from build123d import *

# Parameters (mm, degrees)
F0_R      = 2.25
F1_DEPTH  = 10
F3_DEPTH  = 20
F4_R      = 2.01
F5_DEPTH  = 5
F6_R      = 2.25
F7_DEPTH  = 5
F8_R      = 3.75
F9_DEPTH  = 2
F10_R     = 3.75
F11_DEPTH = 2


with BuildPart() as f1:
    # F0 (on Top) → F1 (new body)
    with BuildSketch(Plane.XY):
        Polygon((15.558824, 6.264706), (15.558824, -35.735294), (35.558824, -35.735294), (35.558824, -13.735294), (55.558824, 6.264706), (120.558824, 6.264706), (120.558824, 26.264706), (35.558824, 26.264706), (35.558824, 6.264706), align=None)
        with Locations((25.558824, -20.735294)):
            Circle(F0_R, mode=Mode.SUBTRACT)
        with Locations((25.558824, -5.735294)):
            Circle(F0_R, mode=Mode.SUBTRACT)
        with Locations((54.558824, 16.264706)):
            Circle(F0_R, mode=Mode.SUBTRACT)
        with Locations((109.558824, 16.264706)):
            Circle(F0_R, mode=Mode.SUBTRACT)
    extrude(amount=F1_DEPTH)

    # F2 (on face) → F3 (join)
    with BuildSketch(Plane.XY.offset(10)):
        Polygon((55.558824, 6.264706), (35.558824, 6.264706), (35.558824, -13.735294), (40.558824, -8.735294), (40.558824, 1.264706), (45.558824, 1.264706), (50.558824, 1.264706), align=None)
    extrude(amount=F3_DEPTH)

    # F4 (on face) → F5 (cut)
    with BuildSketch(Plane(origin=(35.558824, 0, 0), x_dir=(0, -1, 0), z_dir=(-1, 0, 0))):
        with Locations((6.735294, 20)):
            Circle(F4_R)
    extrude(amount=-F5_DEPTH, mode=Mode.SUBTRACT)

    # F6 (on face) → F7 (cut)
    with BuildSketch(Plane(origin=(0, 6.264706, 0), x_dir=(-1, 0, 0), z_dir=(0, 1, 0))):
        with Locations((-48.558824, 20)):
            Circle(F6_R)
    extrude(amount=-F7_DEPTH, mode=Mode.SUBTRACT)

    # F8 (on face) → F9 (cut)
    with BuildSketch(Plane.XZ.offset(-1.264706)):
        with Locations((48.558824, 20)):
            Circle(F8_R)
    extrude(amount=-F9_DEPTH, mode=Mode.SUBTRACT)

    # F10 (on face) → F11 (cut)
    with BuildSketch(Plane.YZ.offset(40.558824)):
        with Locations((-6.735294, 20)):
            Circle(F10_R)
    extrude(amount=-F11_DEPTH, mode=Mode.SUBTRACT)


solid = f1.part
Source: CAD feature listing. Evaluate the final solid. Frame: model axes, mm. A direction names the side the tool comes from. Round coordinates to 2 decimals unless told otherwise and drop trailing zeros. Loops run counter-clockwise (first coordinate to the right, second up) from the corner with the lowest first, then second, coordinate; pieces in that order, holes last.
Q1. Ray query, line 1 (X direction, y = 2.5, z = 20); line 2 (X direction, y = -2.5, z = 21.5); line 3 (Y direction, x = 42, z = 22). Return the intervals inside material, ascending.
Q2. Mould query, pull axis Y, two halves, no side actions, for faces 1 (the face through (50, 3.265, 18)), 2 (the face through (23.31, -5.64, 4.93)), 3 (the face through (37.038, -6.474, 21.993)), 4 (the face through (77, 16, 10)). Classes: pulls with the +Y half, pulls with the -Y half, needs draft (parallel to the pull), parting line crosses it, or undercut.
Q3. First-contact query: P1, Ø6, axis at y = -6.74, z = 20, coming from the -X side; P2, Ø10, axis at x = 42, y = 15.5, coming from the +Z side; P3, Ø11, axis at y = -5, z = 16, coming from the +X side. Flat tips, straight axial feed; report the tip coordinate or a pass-through.
Q4. Section D-D, the plane z = 25.5. Return loops of the section in (x, y).
Q5. Section B-B, the plane y = 17.5. Return loops of the section in (x, z).
Q6. Access query for faces 5 (the face through (44, 1.265, 20)), 6 (the face through (46, 6.265, 20)), 7 (the face through (35.559, -25, 5)). Directions: +Z, -Z, +X, -X, +Y, -Y. A direction counts if a zero-diameter tool reaches every point of the face in a straight line with its end or side. Return the directions, or none.
Q7. Section A-A, the plane x = 109. Return loops of the section in (y, z).
Q8. Section C-C, the plane z = 20. Return loops of the section in (x, y), plus the area to 3 significant figures.
Solutions:
1. line 1: x = 35.56 to 44.81
1. line 2: x = 35.56 to 40.56
1. line 3: y = 1.26 to 6.26
2. face 1: pulls with the -Y half
2. face 2: undercut
2. face 3: undercut
2. face 4: needs draft
3. P1: stops at x = 35.56
3. P2: stops at z = 10
3. P3: stops at x = 40.56
4. outline: (35.56, -13.74) - (40.56, -8.74) - (40.56, 1.26) - (50.56, 1.26) - (55.56, 6.26) - (35.56, 6.26) - close
5. outline: (35.56, 0) - (52.68, 0) - (52.68, 10) - (35.56, 10) - close; (56.44, 0) - (107.68, 0) - (107.68, 10) - (56.44, 10) - close; (111.44, 0) - (120.56, 0) - (120.56, 10) - (111.44, 10) - close
6. face 5: +Z, +X, -Y
6. face 6: +Z, +X, -X, +Y
6. face 7: +Z, -Z, +X, -Y
7. outline: (6.26, 0) - (14.09, 0) - (14.09, 10) - (6.26, 10) - close; (18.44, 0) - (26.26, 0) - (26.26, 10) - (18.44, 10) - close
8. outline: (35.56, -13.74) - (38.81, -10.49) - (38.56, -10.49) - (38.56, -8.75) - (35.56, -8.75) - close; (35.56, -4.73) - (38.56, -4.73) - (38.56, -2.99) - (40.56, -2.99) - (40.56, 1.26) - (44.81, 1.26) - (44.81, 3.26) - (46.31, 3.26) - (46.31, 6.26) - (35.56, 6.26) - close; (50.81, 3.26) - (52.31, 3.26) - (52.31, 3.01) - (55.56, 6.26) - (50.81, 6.26) - close
8. area: 97.5 mm2
